from build123d import *

# Parameters (mm, degrees)
PAD002_DEPTH    = 11
THICKNESS001_T  = 1.5
POCKET006_DEPTH = 20
POCKET007_DEPTH = 32
POCKET009_DEPTH = 5
POCKET014_DEPTH = 5
PAD012_START    = 4.58
PAD012_DEPTH    = 0.92


with BuildPart() as part:
    # Sketch012 → Pad002 (new body)
    with BuildSketch(Plane.XY):
        with BuildLine():
            Line((-19.464986, 23.284984), (-19.464986, 2.515016))
            ThreePointArc((-19.464986, 2.515016), (-17.82478, -1.444793), (-13.864971, -3.085))
            Line((-13.864971, -3.085), (14.264998, -3.085))
            ThreePointArc((14.264998, -3.085), (18.224807, -1.444793), (19.865014, 2.515016))
            Line((19.865014, 2.515016), (19.865014, 23.284984))
            ThreePointArc((19.865014, 23.284984), (18.224807, 27.244793), (14.264998, 28.885))
            Line((14.264998, 28.885), (-13.864971, 28.885))
            ThreePointArc((-13.864971, 28.885), (-17.82478, 27.244793), (-19.464986, 23.284984))
        make_face()
    extrude(amount=PAD002_DEPTH)

    # Thickness001
    thickness001_openings = [part.faces().sort_by_distance(p)[0] for p in [
        (0.200014, 12.9, 0),
    ]]
    offset(amount=THICKNESS001_T, openings=thickness001_openings, kind=Kind.INTERSECTION)

    # Sketch013 → Pocket006 (cut)
    with BuildSketch(Plane.XY):
        with BuildLine():
            Line((-13.664986, -1.535), (11.315014, -1.535))
            ThreePointArc((11.315014, -1.535), (14.320217, -0.290204), (15.565014, 2.715))
            Line((15.565014, 2.715), (15.565014, 23.085))
            ThreePointArc((15.565014, 23.085), (14.320217, 26.090204), (11.315014, 27.335))
            Line((11.315014, 27.335), (-13.664986, 27.335))
            ThreePointArc((-13.664986, 27.335), (-16.67019, 26.090204), (-17.914986, 23.085))
            Line((-17.914986, 23.085), (-17.914986, 2.715))
            ThreePointArc((-17.914986, 2.715), (-16.67019, -0.290204), (-13.664986, -1.535))
        make_face()
    extrude(amount=POCKET006_DEPTH, mode=Mode.SUBTRACT)

    # Sketch018 → Pocket007 (cut)
    with BuildSketch(Plane.XZ):
        with BuildLine():
            Line((-10.6786, 2.39), (-4.2386, 2.39))
            ThreePointArc((-4.2386, 2.39), (-3.213295, 2.814695), (-2.7886, 3.84))
            Line((-2.7886, 3.84), (-2.7886, 4.55))
            ThreePointArc((-2.7886, 4.55), (-3.213295, 5.575305), (-4.2386, 6))
            Line((-4.2386, 6), (-10.6786, 6))
            ThreePointArc((-10.6786, 6), (-11.703905, 5.575305), (-12.1286, 4.55))
            Line((-12.1286, 4.55), (-12.1286, 3.84))
            ThreePointArc((-12.1286, 3.84), (-11.703905, 2.814695), (-10.6786, 2.39))
        make_face()
    extrude(amount=-POCKET007_DEPTH, mode=Mode.SUBTRACT)

    # Sketch022 → Pocket009 (cut)
    with BuildSketch(Plane.XZ):
        with BuildLine():
            Line((-11.864971, 7.25), (-11.864971, 5.75))
            ThreePointArc((-11.864971, 5.75), (-11.572077, 5.042893), (-10.864971, 4.75))
            Line((-10.864971, 4.75), (-6.864971, 4.75))
            ThreePointArc((-6.864971, 4.75), (-6.157864, 5.042893), (-5.864971, 5.75))
            Line((-5.864971, 5.75), (-5.864971, 7.25))
            ThreePointArc((-5.864971, 7.25), (-6.157864, 7.957107), (-6.864971, 8.25))
            Line((-6.864971, 8.25), (-10.864971, 8.25))
            ThreePointArc((-10.864971, 8.25), (-11.572077, 7.957107), (-11.864971, 7.25))
        make_face()
        with BuildLine():
            Line((-3, 7.25), (-3, 5.75))
            ThreePointArc((-3, 5.75), (-2.707107, 5.042893), (-2, 4.75))
            Line((-2, 4.75), (2, 4.75))
            ThreePointArc((2, 4.75), (2.707107, 5.042893), (3, 5.75))
            Line((3, 5.75), (3, 7.25))
            ThreePointArc((3, 7.25), (2.707107, 7.957107), (2, 8.25))
            Line((2, 8.25), (-2, 8.25))
            ThreePointArc((-2, 8.25), (-2.707107, 7.957107), (-3, 7.25))
        make_face()
        with BuildLine():
            Line((6.264998, 7.25), (6.264998, 5.75))
            ThreePointArc((6.264998, 5.75), (6.557891, 5.042893), (7.264998, 4.75))
            Line((7.264998, 4.75), (11.264998, 4.75))
            ThreePointArc((11.264998, 4.75), (11.972105, 5.042893), (12.264998, 5.75))
            Line((12.264998, 5.75), (12.264998, 7.25))
            ThreePointArc((12.264998, 7.25), (11.972105, 7.957107), (11.264998, 8.25))
            Line((11.264998, 8.25), (7.264998, 8.25))
            ThreePointArc((7.264998, 8.25), (6.557891, 7.957107), (6.264998, 7.25))
        make_face()
    extrude(amount=POCKET009_DEPTH, mode=Mode.SUBTRACT)

    # Sketch030 → Pocket014 (cut)
    with BuildSketch(Plane.XZ):
        with BuildLine():
            Line((11.264998, 8.75), (7.264998, 8.75))
            ThreePointArc((7.264998, 8.75), (6.204338, 8.31066), (5.764998, 7.25))
            Line((5.764998, 7.25), (5.764998, 5.75))
            ThreePointArc((5.764998, 5.75), (6.204338, 4.68934), (7.264998, 4.25))
            Line((7.264998, 4.25), (11.264998, 4.25))
            ThreePointArc((11.264998, 4.25), (12.325658, 4.68934), (12.764998, 5.75))
            Line((12.764998, 5.75), (12.764998, 7.25))
            ThreePointArc((12.764998, 7.25), (12.325658, 8.31066), (11.264998, 8.75))
        make_face()
        with BuildLine():
            Line((-12.364971, 7.25), (-12.364971, 5.75))
            ThreePointArc((-12.364971, 5.75), (-11.925631, 4.68934), (-10.864971, 4.25))
            Line((-10.864971, 4.25), (-6.864971, 4.25))
            ThreePointArc((-6.864971, 4.25), (-5.804311, 4.68934), (-5.364971, 5.75))
            Line((-5.364971, 5.75), (-5.364971, 7.25))
            ThreePointArc((-5.364971, 7.25), (-5.804311, 8.31066), (-6.864971, 8.75))
            Line((-6.864971, 8.75), (-10.864971, 8.75))
            ThreePointArc((-10.864971, 8.75), (-11.925631, 8.31066), (-12.364971, 7.25))
        make_face()
        with BuildLine():
            Line((-3.5, 7.25), (-3.5, 5.75))
            ThreePointArc((-3.5, 5.75), (-3.06066, 4.68934), (-2, 4.25))
            Line((-2, 4.25), (2, 4.25))
            ThreePointArc((2, 4.25), (3.06066, 4.68934), (3.5, 5.75))
            Line((3.5, 5.75), (3.5, 7.25))
            ThreePointArc((3.5, 7.25), (3.06066, 8.31066), (2, 8.75))
            Line((2, 8.75), (-2, 8.75))
            ThreePointArc((-2, 8.75), (-3.06066, 8.31066), (-3.5, 7.25))
        make_face()
    extrude(amount=POCKET014_DEPTH, mode=Mode.SUBTRACT)

    # Sketch031 → Pad012 (join)
    with BuildSketch(Plane.XZ.offset(PAD012_START)):
        with BuildLine():
            Line((5.264998, 7.25), (5.264998, 5.75))
            ThreePointArc((5.264998, 5.75), (5.850784, 4.335786), (7.264998, 3.75))
            Line((7.264998, 3.75), (11.264998, 3.75))
            ThreePointArc((11.264998, 3.75), (12.679211, 4.335786), (13.264998, 5.75))
            Line((13.264998, 5.75), (13.264998, 7.25))
            ThreePointArc((13.264998, 7.25), (12.679211, 8.664214), (11.264998, 9.25))
            Line((11.264998, 9.25), (7.264998, 9.25))
            ThreePointArc((7.264998, 9.25), (5.850784, 8.664214), (5.264998, 7.25))
        make_face()
        with BuildLine():
            Line((6.264998, 7.25), (6.264998, 5.75))
            ThreePointArc((6.264998, 5.75), (6.557891, 5.042893), (7.264998, 4.75))
            Line((7.264998, 4.75), (11.264998, 4.75))
            ThreePointArc((11.264998, 4.75), (11.972105, 5.042893), (12.264998, 5.75))
            Line((12.264998, 5.75), (12.264998, 7.25))
            ThreePointArc((12.264998, 7.25), (11.972105, 7.957107), (11.264998, 8.25))
            Line((11.264998, 8.25), (7.264998, 8.25))
            ThreePointArc((7.264998, 8.25), (6.557891, 7.957107), (6.264998, 7.25))
        make_face(mode=Mode.SUBTRACT)
        with BuildLine():
            Line((-12.864971, 7.25), (-12.864971, 5.75))
            ThreePointArc((-12.864971, 5.75), (-12.279184, 4.335786), (-10.864971, 3.75))
            Line((-10.864971, 3.75), (-6.864971, 3.75))
            ThreePointArc((-6.864971, 3.75), (-5.450757, 4.335786), (-4.864971, 5.75))
            Line((-4.864971, 5.75), (-4.864971, 7.25))
            ThreePointArc((-4.864971, 7.25), (-5.450757, 8.664214), (-6.864971, 9.25))
            Line((-6.864971, 9.25), (-10.864971, 9.25))
            ThreePointArc((-10.864971, 9.25), (-12.279184, 8.664214), (-12.864971, 7.25))
        make_face()
        with BuildLine():
            Line((-11.864971, 7.25), (-11.864971, 5.75))
            ThreePointArc((-11.864971, 5.75), (-11.572077, 5.042893), (-10.864971, 4.75))
            Line((-10.864971, 4.75), (-6.864971, 4.75))
            ThreePointArc((-6.864971, 4.75), (-6.157864, 5.042893), (-5.864971, 5.75))
            Line((-5.864971, 5.75), (-5.864971, 7.25))
            ThreePointArc((-5.864971, 7.25), (-6.157864, 7.957107), (-6.864971, 8.25))
            Line((-6.864971, 8.25), (-10.864971, 8.25))
            ThreePointArc((-10.864971, 8.25), (-11.572077, 7.957107), (-11.864971, 7.25))
        make_face(mode=Mode.SUBTRACT)
        with BuildLine():
            Line((-2, 3.75), (2, 3.75))
            ThreePointArc((2, 3.75), (3.414214, 4.335786), (4, 5.75))
            Line((4, 5.75), (4, 7.25))
            ThreePointArc((4, 7.25), (3.414214, 8.664214), (2, 9.25))
            Line((2, 9.25), (-2, 9.25))
            ThreePointArc((-2, 9.25), (-3.414214, 8.664214), (-4, 7.25))
            Line((-4, 7.25), (-4, 5.75))
            ThreePointArc((-4, 5.75), (-3.414214, 4.335786), (-2, 3.75))
        make_face()
        with BuildLine():
            Line((-3, 7.25), (-3, 5.75))
            ThreePointArc((-3, 5.75), (-2.707107, 5.042893), (-2, 4.75))
            Line((-2, 4.75), (2, 4.75))
            ThreePointArc((2, 4.75), (2.707107, 5.042893), (3, 5.75))
            Line((3, 5.75), (3, 7.25))
            ThreePointArc((3, 7.25), (2.707107, 7.957107), (2, 8.25))
            Line((2, 8.25), (-2, 8.25))
            ThreePointArc((-2, 8.25), (-2.707107, 7.957107), (-3, 7.25))
        make_face(mode=Mode.SUBTRACT)
    extrude(amount=PAD012_DEPTH)


with BuildPart() as part_1:
    # Body002 placement: moved
    add(part.part.moved(Location((0, 0, 0.9))))


solid = part_1.part
Could you check a few things on this model? Use its own coordinates, in mm. A direction names the side the tool comes from. Round coordinates to 2 decimals unless told otherwise and drop trailing zeros. Order: outer loops, then holes, each group sorted by start corner. A loop starts at its lowest first (then second) coordinate and runs counter-clockwise, first axis right, second up. Notation, with made-up numbers: M 17.5,28.5 L 59.5,28.5 A32 ccw 59.5,60.5 Z; hole C -3,38.25 d3. An arc over 180 degrees is marked long. One line per item, written item: value.
(1) Imagine slicing it at D-D (x = 8). Write out the boundary of the cut face in (y, z) (3 decimals), and give its area (3 significant figures).
Ans:
outline: M -5.5,4.65 L -4.585,4.65 L -4.585,0.9 L -3.085,0.9 L -3.085,5.15 L -4.58,5.15 L -4.58,5.65 L -5.5,5.65 Z; M -5.5,9.15 L -4.58,9.15 L -4.58,9.65 L -3.085,9.65 L -3.085,11.9 L -1.535,11.9 L -1.535,13.4 L -4.585,13.4 L -4.585,10.15 L -5.5,10.15 Z; M 27.335,11.9 L 28.885,11.9 L 28.885,0.9 L 30.385,0.9 L 30.385,13.4 L 27.335,13.4 Z
area: 37.2 mm^2
(2) Which directions (+Z, -Z, +X, -X, +Y, -Y) give clear straight access to the entire face, cutting with the end or side of a thin tool? Please do faces 1 (the cylindrical face through (-6.15, -5.03, 8.85)), 2 (the flat face through (13.265, -5, 7)), 3 (the flat face through (9, -4, 5.15)).
Ans:
face 1: -Y
face 2: +Z, -Z, +X, -Y
face 3: none
(3) I'm going to push flat-ended pins straight in: P1, Ø1, axis at y = -2, z = 5.5, coming from the -X side; P2, Ø4, axis at x = 17, z = 10, coming from the +Y side; P3, Ø6, axis at y = 26.5, z = 7.5, coming from the +X side; P4, Ø1, axis at x = -15.5, y = -0.5, coming from the +Z side. Where does each tip first touch, or does it pass through?
Ans:
P1: stops at x = -19.72
P2: stops at y = 30.35
P3: stops at x = 21.36
P4: passes through
(4) I need wall thicknesses on line 1 along Y through (x, z) = (-3, 9.5) (3 decimals); line 2 along X through (y, z) = (4, 6.25); line 3 along X through (y, z) = (4, 12.25). Which ranges of each line are inside material? Lowest first, please. Write a range as from..to.
Ans:
line 1: y = -5.5..-3.085, 28.885..30.385
line 2: x = -20.96..-19.46, 19.87..21.37
line 3: x = -20.96..-17.91, 15.57..21.37
(5) Imagine slicing it at C-C (z = 2.25). Write out the boundary of the cut face in (x, y) (3 decimals), and give its area (3 significant figures).
Ans:
outline: M -20.965,2.515 A7.1 ccw -13.865,-4.585 L 14.265,-4.585 A7.1 ccw 21.365,2.515 L 21.365,23.285 A7.1 ccw 14.265,30.385 L -13.865,30.385 A7.1 ccw -20.965,23.285 Z; hole M -19.465,2.515 A5.6 ccw -13.865,-3.085 L 14.265,-3.085 A5.6 ccw 19.865,2.515 L 19.865,23.285 A5.6 ccw 14.265,28.885 L -13.865,28.885 A5.6 ccw -19.465,23.285 Z
area: 207 mm^2
(6) Imagine slicing it at B-B (y = 14.5). Write out the boundary of the cut face in (x, z), and give its area (3 significant figures).
Ans:
outline: M -20.96,0.9 L -19.46,0.9 L -19.46,11.9 L -17.91,11.9 L -17.91,13.4 L -20.96,13.4 Z; M 15.57,11.9 L 19.87,11.9 L 19.87,0.9 L 21.37,0.9 L 21.37,13.4 L 15.57,13.4 Z
area: 46.3 mm^2
(7) Imagine slicing it at A-A (x = -9). Write out the boundary of the cut face in (y, z) (3 decimals).
Ans:
outline: M -5.5,4.65 L -4.585,4.65 L -4.585,0.9 L -3.085,0.9 L -3.085,5.15 L -4.58,5.15 L -4.58,5.65 L -5.5,5.65 Z; M -5.5,9.15 L -4.58,9.15 L -4.58,9.65 L -3.085,9.65 L -3.085,11.9 L -1.535,11.9 L -1.535,13.4 L -4.585,13.4 L -4.585,10.15 L -5.5,10.15 Z; M 27.335,11.9 L 28.885,11.9 L 28.885,6.9 L 30.385,6.9 L 30.385,13.4 L 27.335,13.4 Z; M 28.885,0.9 L 30.385,0.9 L 30.385,3.29 L 28.885,3.29 Z
(8) If we mould it in two halves opening along Y, with no side actions, what happens to faces 4 (the flat face through (0, 30.385, 7)), 5 (the cylindrical face through (14.29, -0.32, 12.64)), 6 (the cylindrical face through (5.866, -5.036, 9.58))? For each: released by +Y, released by -Y, zero draft, split by the parting line, or undercut.
Ans:
face 4: released by +Y
face 5: undercut
face 6: zero draft
